from build123d import *

# Parameters (mm, degrees)
F1_DEPTH    = 45
F2_T1_DEPTH = 45
F3_W        = 4.5
F3_H        = 8.5
F4_DEPTH    = 1.5


# Not quite as in the source:
# - a fillet or chamfer that OpenCascade refuses, or shapes differently, is made with other operations: its cross-section is extruded or revolved along the edge and cut away or added


with BuildPart() as f1:
    # F0 (on Top) → F1 (new body)
    with BuildSketch(Plane.XY):
        Polygon((38, 0), (0, 0), (-38, 0), (-38, 11), (-35, 11), (-35, 12.5), (-39.5, 12.5), (-39.5, -1.5), (-34.25, -1.5), (-32.75, -1.5), (0, -1.5), (32.75, -1.5), (34.25, -1.5), (39.5, -1.5), (39.5, 12.5), (35, 12.5), (35, 11), (38, 11), align=None)
        Polygon((-32.75, -1.5), (-34.25, -1.5), (-34.25, -11.5), (-28.25, -11.5), (-28.25, -10), (-32.75, -10), align=None)
        Polygon((34.25, -11.5), (34.25, -1.5), (32.75, -1.5), (32.75, -10), (28.25, -10), (28.25, -11.5), align=None)
    extrude(amount=F1_DEPTH)

    # F2: fillet of radius 6 on 2 edges, made by hand

    # F2_s2 → F2_t1 (join)
    with BuildSketch(Plane.XY):
        with BuildLine():
            ThreePointArc((-39.5, -1.5), (-35.75, -3.4843134833), (-34.25, -7.4529404499))
            Line((-34.25, -7.4529404499), (-34.25, -1.5))
            Line((-34.25, -1.5), (-39.5, -1.5))
        make_face()
        with BuildLine():
            ThreePointArc((34.25, -7.4529404499), (35.75, -3.4843134833), (39.5, -1.5))
            Line((39.5, -1.5), (34.25, -1.5))
            Line((34.25, -1.5), (34.25, -7.4529404499))
        make_face()
    extrude(amount=F2_T1_DEPTH)

    # F3 (on face) → F4 (join)
    with BuildSketch(Plane(origin=(0, 0, 0), x_dir=(1, 0, 0), z_dir=(0, 0, -1))):
        with BuildLine():
            Line((-32.75, 10), (-28.25, 10))
            Line((-28.25, 10), (-28.25, 11.5))
            Line((-28.25, 11.5), (-34.25, 11.5))
            Line((-34.25, 11.5), (-34.25, 7.4529404499))
            ThreePointArc((-34.25, 7.4529404499), (-35.75, 3.4843134833), (-39.5, 1.5))
            Line((-39.5, 1.5), (-39.5, -12.5))
            Line((-39.5, -12.5), (-35, -12.5))
            Line((-35, -12.5), (-35, -11))
            Line((-35, -11), (-38, -11))
            Line((-38, -11), (-38, 0))
            Line((-38, 0), (-29.5, 0))
            Line((-29.5, 0), (21.5, 0))
            Line((21.5, 0), (38, 0))
            Line((38, 0), (38, -11))
            Line((38, -11), (35, -11))
            Line((35, -11), (35, -12.5))
            Line((35, -12.5), (39.5, -12.5))
            Line((39.5, -12.5), (39.5, 1.5))
            ThreePointArc((39.5, 1.5), (35.75, 3.4843134833), (34.25, 7.4529404499))
            Line((34.25, 7.4529404499), (34.25, 11.5))
            Line((34.25, 11.5), (28.25, 11.5))
            Line((28.25, 11.5), (28.25, 10))
            Line((28.25, 10), (32.75, 10))
            Line((32.75, 10), (32.75, 1.5))
            Line((32.75, 1.5), (28.25, 1.5))
            Line((28.25, 1.5), (-28.25, 1.5))
            Line((-28.25, 1.5), (-32.75, 1.5))
            Line((-32.75, 1.5), (-32.75, 10))
        make_face()
        with Locations((-30.5, 5.75)):
            Rectangle(F3_W, F3_H)
        Polygon((-35, -11), (-35, -12.5), (-29.5, -12.5), (-29.5, 0), (-38, 0), (-38, -11), align=None)
        with Locations((30.5, 5.75)):
            Rectangle(F3_W, F3_H)
        Polygon((21.5, -12.5), (35, -12.5), (35, -11), (38, -11), (38, 0), (21.5, 0), align=None)
    extrude(amount=F4_DEPTH)


solid = f1.part
Read the model definition and answer for the solid it produces. Units are mm, in the model's axes. A direction names the side the tool comes from. Round coordinates to 2 decimals unless told otherwise and drop trailing zeros. Write each loop counter-clockwise with the first axis right and the second up, starting at its lowest first coordinate (ties: lowest second). Pieces come first, ordered by that corner, then holes.
Q1. Find section A-A on y = 8.75. Determine the outline of the cut face in (x, z).
Values:
outline: (-39.5, -1.5) - (-29.5, -1.5) - (-29.5, 0) - (-38, 0) - (-38, 45) - (-39.5, 45) - close; (21.5, -1.5) - (39.5, -1.5) - (39.5, 45) - (38, 45) - (38, 0) - (21.5, 0) - close
Q2. Flat-ended cylindrical pins translate along their axes: P1, Ø2, axis at x = -30, y = -7, coming from the +Z side; P2, Ø8, axis at y = -5, z = 21, coming from the -X side; P3, Ø3, axis at y = -9.5, z = 31.5, coming from the +X side; P4, Ø14, axis at x = 13.5, z = 26, coming from the -Y side. Find the tip coordinate at first contact, or state that the pin passes through.
Values:
P1: stops at z = 0
P2: stops at x = -39.5
P3: stops at x = 34.25
P4: stops at y = -1.5
Q3. The mould has two halves that part along X. Classify faces 1 (the face through (-34.25, -10, 22)), 2 (the face through (-1, 0, 22)), 3 (the face through (39.5, 6, 22)): released by +X, released by -X, zero draft, split by the parting line, or undercut.
Values:
face 1: released by -X
face 2: undercut
face 3: released by +X
Q4. Find section D-D on x = -2. Determine the outline of the cut face in (y, z), and give its area (4 significant figures).
Values:
outline: (-1.5, -1.5) - (0, -1.5) - (0, 45) - (-1.5, 45) - close
area: 69.75 mm2
Q5. Straight lines are drawn through the part: line 1 (X direction, y = 5.25, z = 29); line 2 (Y direction, x = 29, z = 36.5); line 3 (Y direction, x = 1.5, z = 3.5). For each, find the intervals that lie inside material, in ascending order.
Values:
line 1: x = -39.5 to -38, 38 to 39.5
line 2: y = -11.5 to -10, -1.5 to 0
line 3: y = -1.5 to 0
Q6. Find section C-C on y = -6.5. Determine the outline of the cut face in (x, z), and give its area (3 significant figures).
Values:
outline: (-34.33, -1.5) - (-28.25, -1.5) - (-28.25, 0) - (-32.75, 0) - (-32.75, 45) - (-34.33, 45) - close; (28.25, -1.5) - (34.33, -1.5) - (34.33, 45) - (32.75, 45) - (32.75, 0) - (28.25, 0) - close
area: 160 mm2
Q7. Find section B-B on z = 29. Determine the outline of the cut face in (x, y), and give its area (3 significant figures).
Values:
outline: (-39.5, -1.5) arc R6 cw to (-34.25, -7.45) - (-34.25, -11.5) - (-28.25, -11.5) - (-28.25, -10) - (-32.75, -10) - (-32.75, -1.5) - (32.75, -1.5) - (32.75, -10) - (28.25, -10) - (28.25, -11.5) - (34.25, -11.5) - (34.25, -7.45) arc R6 cw to (39.5, -1.5) - (39.5, 12.5) - (35, 12.5) - (35, 11) - (38, 11) - (38, 0) - (-38, 0) - (-38, 11) - (-35, 11) - (-35, 12.5) - (-39.5, 12.5) - close
area: 223 mm2
Q8. A tool of negligible diameter and unlimited length cuts with its end or side. For faces 4 (the face through (36, 12.5, 20)), 5 (the face through (31, -11.5, 22)), 6 (the face through (-35, 12, 22)), 7 (the face through (-37, 11, 22)), 8 (the face through (28.25, -11, 17)), from which of +Z, -Z, +X, -X, +Y, -Y can it reach the whole face along a straight path? Write none if from no direction.
Values:
face 4: +Z, -Z, +X, -X, +Y
face 5: +Z, -Z, +X, -X, -Y
face 6: +Z, +Y
face 7: +Z
face 8: +Z, -Z, -Y
